Build history of the part. All positions in model axes, mm. A direction names the side the tool comes from. Give positions to 0.01 mm unless a question says otherwise; leave off trailing zeros. Loops run counter-clockwise (first coordinate to the right, second up) from the corner with the lowest first, then second, coordinate; pieces in that order, holes last. Notation, with made-up numbers: M -35,-32 L -14,-32 A20 ccw -14,-8 Z; hole C 37.5,75 d11. An arc over 180 degrees is marked long. Answer as a JSON object with one key per item and string values. Group by question number.
1. Drop flat-ended pins along their axis: pin 1 Ø1.8 at (x, y) = (-3.736, 13.59) entering from +Z; pin 2 Ø3.5 at (x, z) = (41, -3.5) entering from +Y; pin 3 Ø3.5 at (y, z) = (-2, 1) entering from -X; pin 4 Ø4.5 at (x, z) = (46.276, -3.475) entering from -Y. Give the stop position or say it passes through.
2. Drill centre lines: line 1 along Y through (x, z) = (43, -1); line 2 along Y through (x, z) = (22.5, 2.5); line 3 along Z through (x, y) = (13, 2) (3 decimals). Where is each one in solid material? Low to high. Write a range as [from, to].
3. Slice it at D-D (x = 26.5). List the corners of the cut face in (y, z) (3 decimals), then the cut area to 3 significant figures.
4. Mould opens along X. For faces 1 (the face through (49.751, -6, 1)), 2 (the face through (44, -10.8, -3)), 3 (the face through (44.345, 4.88, 1.565)) say: released by +X, released by -X, zero draft, split by the parting line, or undercut.
5. Slice it at C-C (x = 38.5). List the corners of the cut face in (y, z) (3 decimals), then the cut area to 3 significant figures.
6. Slice it at A-A (y = -12.3). Give the number of separate pieces and of enclosed holes in the cut face, then the cut area to 3 significant figures.
7. Slice it at B-B (y = 4). List the corners of the cut face in (x, z) (3 decimals), then the cut area to 3 significant figures.
8. 3-axis set-ups, long thin cutter, end or side, ignore diameter. For faces 4 (the face through (17, 14.8, 2)), 5 (the face through (-6.416, -2, 2)), 6 (the face through (27.5, -14.8, 0.3)): which of +Z, -Z, +X, -X, +Y, -Y reach the whole face in a straight line?
from build123d import *

# Parameters (mm, degrees)
SKETCH1_W            = 6.266
SKETCH1_H            = 19.6
SKETCH1_R            = 1.675
SKETCH1_W_2          = 52.832
SKETCH1_H_2          = 5
BOSS_EXTRUDE2_DEPTH  = 3.175
SKETCH3_W            = 30
SKETCH3_H            = 29.6
BOSS_EXTRUDE3_DEPTH  = 3.175
SKETCH4_R            = 4.75
CUT_EXTRUDE1_DEPTH   = 10
BOSS_EXTRUDE14_DEPTH = 3.175
CUT_EXTRUDE8_DEPTH   = 10
SKETCH24_R           = 1.675
CUT_EXTRUDE9_DEPTH   = 10
SKETCH25_R           = 3.675
SKETCH25_R_2         = 1.675
BOSS_EXTRUDE15_DEPTH = 3.175
SKETCH27_W           = 52.932563224
SKETCH27_H           = 23.005559857
BOSS_EXTRUDE16_DEPTH = 3.175
CUT_EXTRUDE14_DEPTH  = 10
SKETCH29_R           = 1.675
CUT_EXTRUDE15_DEPTH  = 10
SKETCH30_R           = 1.475
CUT_EXTRUDE16_DEPTH  = 10
SKETCH31_R           = 3.675
SKETCH31_R_2         = 1.675
BOSS_EXTRUDE17_DEPTH = 3.175
SKETCH33_R           = 1.475
CUT_EXTRUDE17_DEPTH  = 53.757206626
SKETCH37_R           = 3.475
SKETCH37_R_2         = 1.475
BOSS_EXTRUDE21_DEPTH = 4
BOSS_EXTRUDE22_DEPTH = 4
SKETCH39_R           = 1.675
SKETCH39_R_2         = 1.475
BOSS_EXTRUDE23_DEPTH = 3.175


with BuildPart() as part:
    # Sketch1 → Boss-Extrude2 (new body)
    # profile 1 of 4: a face of its own
    with BuildSketch(Plane.XY):
        with Locations((-23.283, 0)):
            Rectangle(SKETCH1_W, SKETCH1_H)
        with Locations((-23.95, -4.974)):
            Circle(SKETCH1_R, mode=Mode.SUBTRACT)
        with Locations((-23.95, 4.974)):
            Circle(SKETCH1_R, mode=Mode.SUBTRACT)
    # profile 2 of 4: a face of its own
    with BuildSketch(Plane.XY):
        with Locations((0, -12.3)):
            Rectangle(SKETCH1_W_2, SKETCH1_H_2)
    # profile 3 of 4: a face of its own
    with BuildSketch(Plane.XY):
        with Locations((0, 12.3)):
            Rectangle(SKETCH1_W_2, SKETCH1_H_2)
    # profile 4 of 4: a face of its own
    with BuildSketch(Plane.XY):
        with Locations((23.283, 0)):
            Rectangle(SKETCH1_W, SKETCH1_H)
        with Locations((23.95, -4.974)):
            Circle(SKETCH1_R, mode=Mode.SUBTRACT)
        with Locations((23.95, 4.974)):
            Circle(SKETCH1_R, mode=Mode.SUBTRACT)
    extrude(amount=BOSS_EXTRUDE2_DEPTH)

    # Sketch3 → Boss-Extrude3 (add)
    with BuildSketch(Plane.XY.offset(3.175)):
        with Locations((41.416, 0)):
            Rectangle(SKETCH3_W, SKETCH3_H)
    extrude(amount=-BOSS_EXTRUDE3_DEPTH)

    # Sketch4 → Cut-Extrude1 (cut)
    with BuildSketch(Plane(origin=(0, 0, 0), x_dir=(-1, 0, 0), z_dir=(0, 0, -1))):
        with Locations((-40.576, 7.77)):
            Circle(SKETCH4_R)
    extrude(amount=-CUT_EXTRUDE1_DEPTH, mode=Mode.SUBTRACT)

    # Sketch22 → Boss-Extrude14 (add)
    with BuildSketch(Plane(origin=(0, 0, 0), x_dir=(-1, 0, 0), z_dir=(0, 0, -1))):
        with BuildLine():
            ThreePointArc((-34.680262133, 14.8), (-40.576, 16.945), (-46.471737867, 14.8))
            Line((-46.471737867, 14.8), (-34.680262133, 14.8))
        make_face()
    extrude(amount=-BOSS_EXTRUDE14_DEPTH)

    # Sketch23 → Cut-Extrude8 (cut)
    with BuildSketch(Plane(origin=(0, 0, 0), x_dir=(-1, 0, 0), z_dir=(0, 0, -1))):
        with BuildLine():
            Line((-49.751, -14.8), (-49.751, 7.77))
            ThreePointArc((-49.751, 7.77), (-48.890866804, 11.648609936), (-46.471737867, 14.8))
            Line((-46.471737867, 14.8), (-56.416, 14.8))
            Line((-56.416, 14.8), (-56.416, -14.8))
            Line((-56.416, -14.8), (-49.751, -14.8))
        make_face()
    extrude(amount=-CUT_EXTRUDE8_DEPTH, mode=Mode.SUBTRACT)

    # Sketch24 → Cut-Extrude9 (cut)
    with BuildSketch(Plane(origin=(0, 0, 0), x_dir=(-1, 0, 0), z_dir=(0, 0, -1))):
        with Locations((23.736, 13.59)):
            Circle(SKETCH24_R)
    extrude(amount=-CUT_EXTRUDE9_DEPTH, mode=Mode.SUBTRACT)

    # Sketch25 → Boss-Extrude15 (add)
    # profile 1 of 3: a face of its own
    with BuildSketch(Plane(origin=(0, 0, 0), x_dir=(-1, 0, 0), z_dir=(0, 0, -1))):
        with Locations((23.95, -4.974)):
            Circle(SKETCH25_R)
        with Locations(Location((23.95, -4.974, 0), (0, 0, 180))):
            Circle(SKETCH25_R_2, mode=Mode.SUBTRACT)
    # profile 2 of 3: a face of its own
    with BuildSketch(Plane(origin=(0, 0, 0), x_dir=(-1, 0, 0), z_dir=(0, 0, -1))):
        with Locations((23.95, 4.974)):
            Circle(SKETCH25_R)
        with Locations(Location((23.95, 4.974, 0), (0, 0, 180))):
            Circle(SKETCH25_R_2, mode=Mode.SUBTRACT)
    # profile 3 of 3: a face of its own
    with BuildSketch(Plane(origin=(0, 0, 0), x_dir=(-1, 0, 0), z_dir=(0, 0, -1))):
        with Locations((23.736, 13.59)):
            Circle(SKETCH25_R)
        with Locations((23.736, 13.59)):
            Circle(SKETCH25_R_2, mode=Mode.SUBTRACT)
    extrude(amount=-BOSS_EXTRUDE15_DEPTH)

    # Sketch27 → Boss-Extrude16 (add)
    with BuildSketch(Plane(origin=(0, 0, 0), x_dir=(-1, 0, 0), z_dir=(0, 0, -1))):
        with Locations((-0.417160697, -0.481381251)):
            Rectangle(SKETCH27_W, SKETCH27_H)
    extrude(amount=-BOSS_EXTRUDE16_DEPTH)

    # Sketch28 → Cut-Extrude14 (cut)
    with BuildSketch(Plane(origin=(0, 0, 0), x_dir=(-1, 0, 0), z_dir=(0, 0, -1))):
        Polygon((26.416, 8.97792488), (26.416, -8.885991227), (33.695668031, -3.414754928), align=None)
    extrude(amount=-CUT_EXTRUDE14_DEPTH, mode=Mode.SUBTRACT)

    # Sketch29 → Cut-Extrude15 (cut)
    # profile 1 of 4: a face of its own
    with BuildSketch(Plane(origin=(0, 0, 0), x_dir=(-1, 0, 0), z_dir=(0, 0, -1))):
        with BuildLine():
            Line((6.416, -14.8), (26.416, -14.8))
            Line((26.416, -14.8), (26.416, 8.759294646))
            Line((26.416, 8.759294646), (26.416, 11.075397646))
            Line((26.416, 11.075397646), (26.416, 16.104602354))
            ThreePointArc((26.416, 16.104602354), (22.973400892, 17.185005925), (20.265909944, 14.8))
            Line((20.265909944, 14.8), (6.416, 14.8))
            Line((6.416, 14.8), (6.416, -14.8))
        make_face()
        with Locations((23.736, 13.59)):
            Circle(SKETCH29_R, mode=Mode.SUBTRACT)
    # profile 2 of 4: a face of its own
    with BuildSketch(Plane(origin=(0, 0, 0), x_dir=(-1, 0, 0), z_dir=(0, 0, -1))):
        with BuildLine():
            Line((26.416, 11.075397646), (26.416, 8.759294646))
            Line((26.416, 8.759294646), (29.849387413, 8.759294646))
            Line((29.849387413, 8.759294646), (29.849387413, 20.986227432))
            Line((29.849387413, 20.986227432), (26.416, 20.986227432))
            Line((26.416, 20.986227432), (26.416, 16.104602354))
            ThreePointArc((26.416, 16.104602354), (27.411, 13.59), (26.416, 11.075397646))
        make_face()
    # profile 3 of 4: a face of its own
    with BuildSketch(Plane(origin=(0, 0, 0), x_dir=(-1, 0, 0), z_dir=(0, 0, -1))):
        with BuildLine():
            Line((26.416, 16.104602354), (26.416, 11.075397646))
            ThreePointArc((26.416, 11.075397646), (27.411, 13.59), (26.416, 16.104602354))
        make_face()
    # profile 4 of 4: a face of its own
    with BuildSketch(Plane(origin=(0, 0, 0), x_dir=(-1, 0, 0), z_dir=(0, 0, -1))):
        with BuildLine():
            Line((6.416, 20.986227432), (6.416, 14.8))
            Line((6.416, 14.8), (20.265909944, 14.8))
            ThreePointArc((20.265909944, 14.8), (22.973400892, 17.185005925), (26.416, 16.104602354))
            Line((26.416, 16.104602354), (26.416, 20.986227432))
            Line((26.416, 20.986227432), (6.416, 20.986227432))
        make_face()
    extrude(amount=-CUT_EXTRUDE15_DEPTH, mode=Mode.SUBTRACT)

    # Sketch30 → Cut-Extrude16 (cut)
    with BuildSketch(Plane(origin=(0, 0, 0), x_dir=(-1, 0, 0), z_dir=(0, 0, -1))):
        with Locations((3.736, 13.59)):
            Circle(SKETCH30_R)
    extrude(amount=-CUT_EXTRUDE16_DEPTH, mode=Mode.SUBTRACT)

    # Sketch31 → Boss-Extrude17 (add)
    with BuildSketch(Plane(origin=(0, 0, 0), x_dir=(-1, 0, 0), z_dir=(0, 0, -1))):
        with Locations((3.736, 13.59)):
            Circle(SKETCH31_R)
        with Locations((3.736, 13.59)):
            Circle(SKETCH31_R_2, mode=Mode.SUBTRACT)
    extrude(amount=-BOSS_EXTRUDE17_DEPTH)

    # Sketch33 → Cut-Extrude17 (cut, through all)
    with BuildSketch(Plane(origin=(0, 0, 0), x_dir=(-1, 0, 0), z_dir=(0, 0, -1))):
        with Locations((3.741, -12.3)):
            Circle(SKETCH33_R)
    extrude(amount=-CUT_EXTRUDE17_DEPTH, mode=Mode.SUBTRACT)

    # Sketch37 → Boss-Extrude21 (add)
    # profile 1 of 3: a face of its own
    with BuildSketch(Plane(origin=(0, -14.8, 0), x_dir=(-1, 0, 0), z_dir=(0, -1, 0))):
        with BuildLine():
            ThreePointArc((-46.276, 0), (-48.733196065, 1.017803935), (-49.751, 3.475))
            Line((-49.751, 3.475), (-49.751, 0))
            Line((-49.751, 0), (-46.276, 0))
        make_face()
    # profile 2 of 3: a face of its own
    with BuildSketch(Plane(origin=(0, -14.8, 0), x_dir=(-1, 0, 0), z_dir=(0, -1, 0))):
        with Locations((-46.276, 3.475)):
            Circle(SKETCH37_R)
        with Locations(Location((-46.276, 3.475, 0), (0, 0, 180))):
            Circle(SKETCH37_R_2, mode=Mode.SUBTRACT)
    # profile 3 of 3: a face of its own
    with BuildSketch(Plane(origin=(0, -14.8, 0), x_dir=(-1, 0, 0), z_dir=(0, -1, 0))):
        with BuildLine():
            Line((-42.801, 0), (-42.801, 3.475))
            ThreePointArc((-42.801, 3.475), (-43.818803935, 1.017803935), (-46.276, 0))
            Line((-46.276, 0), (-42.801, 0))
        make_face()
    extrude(amount=-BOSS_EXTRUDE21_DEPTH)

    # Sketch38 → Boss-Extrude22 (add)
    with BuildSketch(Plane(origin=(0, -14.8, 0), x_dir=(-1, 0, 0), z_dir=(0, -1, 0))):
        with BuildLine():
            Line((-35.826, 0), (-42.801, 0))
            Line((-42.801, 0), (-42.801, 3.475))
            Line((-42.801, 3.475), (-46.276, 6.95))
            ThreePointArc((-46.276, 6.95), (-40.28432198, 4.627774865), (-35.826, 0))
        make_face()
    extrude(amount=-BOSS_EXTRUDE22_DEPTH)

    # Sketch39 → Boss-Extrude23 (add)
    with BuildSketch(Plane(origin=(0, 0, 0), x_dir=(-1, 0, 0), z_dir=(0, 0, -1))):
        with Locations((3.736, 13.59)):
            Circle(SKETCH39_R)
        with Locations((3.736, 13.59)):
            Circle(SKETCH39_R_2, mode=Mode.SUBTRACT)
    extrude(amount=-BOSS_EXTRUDE23_DEPTH)


solid = part.part
Established:
{
 "1": {"pin 1": "passes through", "pin 2": "stops at y = -10.8", "pin 3": "stops at x = -6.42", "pin 4": "stops at y = -14.8"},
 "2": {"line 1": "y = [-14.8, -10.8]", "line 2": "y = [-14.8, 14.8]", "line 3": "z = [0, 3.175]"},
 "3": {"outline": "M -14.8,0 L 14.8,0 L 14.8,3.175 L -14.8,3.175 Z", "area": "94.0 mm^2"},
 "4": {"face 1": "released by +X", "face 2": "zero draft", "face 3": "undercut"},
 "5": {"outline": "M -14.8,-3.235 L -10.8,-3.235 L -10.8,0 L 3.498,0 L 3.498,3.175 L -14.8,3.175 Z; M 12.042,0 L 16.707,0 L 16.707,3.175 L 12.042,3.175 Z", "area": "85.8 mm^2"},
 "6": {"separate pieces": "2", "enclosed holes": "1", "area": "232 mm^2"},
 "7": {"outline": "M -6.416,0 L 37.686,0 L 37.686,3.175 L -6.416,3.175 Z; M 43.466,0 L 49.751,0 L 49.751,3.175 L 43.466,3.175 Z", "area": "160 mm^2"},
 "8": {"face 4": "+Z, -Z, +Y", "face 5": "+Z, -Z, -X, -Y", "face 6": "+Z, -Z, +X, -X, -Y"}
}
